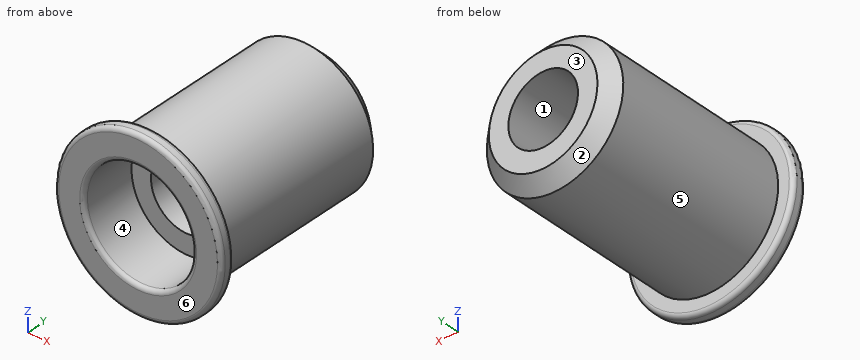
from build123d import *

# Parameters (mm, degrees)
ESBO_O1_R                     = 3
EXTRUS_O1_DEPTH               = 0.5
ESBO_O2_R                     = 2.45
EXTRUS_O2_DEPTH               = 7
CHANFRO1_SIZE                 = 0.5
ESBO_O3_R                     = 1.95
EXTRUS_O3_DEPTH               = 2
ESBO_O4_R                     = 1.05
EXTRUS_O4_DEPTH               = 10
FURO_ROSCADO_DE_M3X0_53_D     = 2.5
FURO_ROSCADO_DE_M3X0_53_DEPTH = 8.5
FURO_ROSCADO_DE_M3X0_53_TIP   = 0.751075774
FILETE1_R                     = 0.15


with BuildPart() as part:
    # Esboço1 → Extrusão1 (new body)
    with BuildSketch(Plane(origin=(0, 0, 0), x_dir=(1, 0, 0), z_dir=(0, 1, 0))):
        with Locations(Location((-26.751205923, -11.338633094, 0), (0, 0, 270))):
            Circle(ESBO_O1_R)
    extrude(amount=EXTRUS_O1_DEPTH)

    # Esboço2 → Extrusão2 (add)
    with BuildSketch(Plane(origin=(0, 0.5, 0), x_dir=(1, 0, 0), z_dir=(0, 1, 0))):
        with Locations(Location((-26.751205923, -11.338633094, 0), (0, 0, 270))):
            Circle(ESBO_O2_R)
    extrude(amount=EXTRUS_O2_DEPTH)

    # Chanfro1
    chanfro1_edges = [part.edges().sort_by_distance(p)[0] for p in [
        (-26.751205923, 7.5, 8.888633094),
    ]]
    chamfer(chanfro1_edges, length=CHANFRO1_SIZE)

    # Esboço3 → Extrusão3 (cut)
    with BuildSketch(Plane.XZ):
        with Locations(Location((-26.751205923, 11.338633094, 0), (0, 0, 270))):
            Circle(ESBO_O3_R)
    extrude(amount=-EXTRUS_O3_DEPTH, mode=Mode.SUBTRACT)

    # Esboço4 → Extrusão4 (cut)
    with BuildSketch(Plane(origin=(0, 7.5, 0), x_dir=(1, 0, 0), z_dir=(0, 1, 0))):
        with Locations(Location((-26.751205923, -11.338633094, 0), (0, 0, 270))):
            Circle(ESBO_O4_R)
    extrude(amount=-EXTRUS_O4_DEPTH, mode=Mode.SUBTRACT)

    # Furo roscado de M3x0.53
    with Locations(Plane(origin=(-26.751205923, 7.5, 11.338633094), x_dir=(0, 0, 1), z_dir=(0, 1, 0))):
        with Locations((0, 0)):
            Hole(FURO_ROSCADO_DE_M3X0_53_D / 2, depth=FURO_ROSCADO_DE_M3X0_53_DEPTH)
            with Locations((0, 0, -(FURO_ROSCADO_DE_M3X0_53_DEPTH + FURO_ROSCADO_DE_M3X0_53_TIP / 2))):  # 118° drill point
                Cone(0, FURO_ROSCADO_DE_M3X0_53_D / 2, FURO_ROSCADO_DE_M3X0_53_TIP, mode=Mode.SUBTRACT)

    # Filete1
    filete1_edges = [part.edges().sort_by_distance(p)[0] for p in [
        (-26.751205923, 0, 13.288633094),
        (-26.751205923, 0, 8.338633094),
        (-26.751205923, 0.5, 8.338633094),
    ]]
    fillet(filete1_edges, radius=FILETE1_R)


solid = part.part
Design review of the part built by this model. Coordinates are the model's own, in mm. Face numbers are marked on the shaded views. A direction names the side the tool comes from. Round coordinates to 2 decimals unless told otherwise and drop trailing zeros. Write each loop counter-clockwise with the first axis right and the second up, starting at its lowest first coordinate (ties: lowest second). Pieces come first, ordered by that corner, then holes.
Item 1: Consider section A-A on y = 3.5. Give the boundary of the cut face in (x, z).
Item 2: For the marked faces 4, 5 and 6, list the 3-axis set-ups (+Z, -Z, +X, -X, +Y, -Y) from which the entire face can be reached by the end or side of a thin tool; tool diameter is ignored.
Item 3: Wall thickness on L1, parallel to X at y = 6, z = 11.25; L2, parallel to Z at x = -27.75, y = 1.25; L3, parallel to Y at x = -26.5, z = 10: over which ranges is each line inside the solid? List them lowest first.
Item 4: Consider section B-B on y = 1.75. Give the boundary of the cut face in (x, z).
Item 5: For pin 1 Ø2 at (x, z) = (-24.5, 9) entering from +Y; pin 2 Ø1.5 at (y, z) = (5.5, 10.5) entering from +X; pin 3 Ø1.5 at (x, y) = (-25, 5.5) entering from +Z, all flat-tipped, find the tip position at first contact; note any pin that passes through.
Item 6: Draft analysis for pull direction X (two halves, no side actions). For the marked faces 1, 2 and 3, state which applies: released by +X, released by -X, zero draft, split by the parting line, or undercut.
Check values:
1. outline: circle Ø4.9 at (-26.75, 11.34); hole circle Ø2.5 at (-26.75, 11.34)
2. face 4: -Y
2. face 5: +Y
2. face 6: +Z, -Z, +X, -X, -Y
3. L1: x = -29.2 to -28, -25.5 to -24.3
3. L2: z = 9.1 to 9.66, 13.01 to 13.58
3. L3: y = 2 to 7.5
4. outline: circle Ø4.9 at (-26.75, 11.34); hole circle Ø3.9 at (-26.75, 11.34)
5. pin 1: stops at y = 7.2
5. pin 2: stops at x = -24.3
5. pin 3: stops at z = 13.57
6. face 1: undercut
6. face 2: split by the parting line
6. face 3: zero draft
